Autodesk Inventor part; units mm, degrees
ref_plane "YZ Plane" through (0, 0, 0) normal (1, 0, 0) x (0, 1, 0)
ref_plane "XZ Plane" through (0, 0, 0) normal (0, 1, 0) x (-1, 0, 0)
ref_plane "XY Plane" through (0, 0, 0) normal (0, 0, 1) x (1, 0, 0)
sketch "Boceto1" plane through (0, 0, 0) normal (0, 0, 1) x (1, 0, 0)
  line L0 (0.1195, 0.0416) -> (6.4695, 0.0416)
  line L1 (6.4695, 0.0416) -> (6.4695, 19.0916)
  line L2 (6.4695, 19.0916) -> (0.1195, 19.0916)
  line L3 (0.1195, 19.0916) -> (0.1195, 0.0416)
  line L4 (6.4695, 0.0416) -> (20.6935, 0.0416)
  line L5 (20.6935, 0.0416) -> (20.6935, 26.2036)
  line L6 (20.6935, 26.2036) -> (6.4695, 26.2036)
  line L7 (6.4695, 26.2036) -> (6.4695, 0.0416)
  line L8 (20.6935, 0.0416) -> (30.3455, 0.0416)
  line L9 (30.3455, 0.0416) -> (30.3455, 22.3936)
  line L10 (30.3455, 22.3936) -> (20.6935, 22.3936)
  line L11 (20.6935, 22.3936) -> (20.6935, 0.0416)
  line L12 (30.3455, 0.0416) -> (44.5695, 0.0416)
  line L13 (44.5695, 0.0416) -> (44.5695, 26.2036)
  line L14 (44.5695, 26.2036) -> (30.3455, 26.2036)
  line L15 (30.3455, 26.2036) -> (30.3455, 0.0416)
  line L16 (44.5695, 0.0416) -> (50.9195, 0.0416)
  line L17 (50.9195, 0.0416) -> (50.9195, 19.0916)
  line L18 (50.9195, 19.0916) -> (44.5695, 19.0916)
  line L19 (44.5695, 19.0916) -> (44.5695, 0.0416)
  line L20 (0.1195, 0.0416) -> (50.9195, 0.0416)
  dimension "d2" = 19.05
  dimension "d3" = 26.162
  dimension "d4" = 9.652
  dimension "d5" = 50.8
  dimension "d6" = 14.224
  dimension "d7" = 6.35
  dimension "d8" = 3.81
revolve "Revolución1" add sketch "Boceto1" angle 360 about axis through (0.1195, 0.0416, 0) along (1, 0, 0)
sketch "Boceto2" plane through (0.1195, 0.0416, 0) normal (-1, 0, 0) x (0, 0, 1)
  circle A0 centre (0, -0.0416) radius 10.9883
extrude "Extrusión1" cut sketch "Boceto2" against normal blind 50.8
equation "\"d2\" = 0.5 * DistC"
equation "\"d3\" = 0.5 * DistA"
equation "\"d4\" = DistE"
equation "\"d5\" = DistB"
equation "\"d6\" = DistX"
equation "\"d7\" = DistD - DistX"
equation "\"d10\" = DistB"
equation "\"DistA\" = 52.324"
equation "\"DistB\" = 50.8"
equation "\"DistC\" = 38.1"
equation "\"DistD\" = 20.574"
equation "\"DistE\" = 9.652"
equation "\"DistX\" = 14.224"
properties part number "Pieza2-Tarea2"
Build history of the part. All positions in model axes, mm. A direction names the side the tool comes from. Round coordinates to 2 decimals unless told otherwise and drop trailing zeros. Order: outer loops, then holes, each group sorted by start corner. A loop starts at its lowest first (then second) coordinate and runs counter-clockwise, first axis right, second up. Notation, with made-up numbers: (2.5, 66) -> (51.5, 66) arc R19 cw to (51.5, 73) -> close; hole circle Ø11 at (-34, 6). An arc over 180 degrees is marked (long way). Answer in a Markdown table with one row per item.
1) Wall check: L1, parallel to X at y = 24.5, z = -1.5; L2, parallel to Y at x = 25, z = -0.5; L3, parallel to Z at x = 36, y = -0.5. Give the ranges that are in metal, low to high.
Values:
| item | result |
|---|---|
| L1 | 6.47 to 20.69, 30.35 to 44.57 |
| L2 | -22.3 to -10.98, 10.98 to 22.39 |
| L3 | -26.16 to -10.98, 10.98 to 26.16 |
2) Mould opens along Z. For faces 6 (the cylindrical face through (25.16, 3.3, 10.48)), 7 (the cylindrical face through (37.358, 24.995, -7.858)), 8 (the flat face through (0.12, 8, -8)) say: released by +Z, released by -Z, zero draft, split by the parting line, or undercut.
Values:
| item | result |
|---|---|
| face 6 | undercut |
| face 7 | split by the parting line |
| face 8 | zero draft |
3) Band-saw the part on B-B on y = 0. Give the cut face in (x, z).
Values:
| item | result |
|---|---|
| outline | (0.12, -19.05) -> (6.47, -19.05) -> (6.47, -26.16) -> (20.69, -26.16) -> (20.69, -22.35) -> (30.35, -22.35) -> (30.35, -26.16) -> (44.57, -26.16) -> (44.57, -19.05) -> (50.92, -19.05) -> (50.92, -10.99) -> (0.12, -10.99) -> close; (0.12, 10.99) -> (50.92, 10.99) -> (50.92, 19.05) -> (44.57, 19.05) -> (44.57, 26.16) -> (30.35, 26.16) -> (30.35, 22.35) -> (20.69, 22.35) -> (20.69, 26.16) -> (6.47, 26.16) -> (6.47, 19.05) -> (0.12, 19.05) -> close |
4) Band-saw the part on D-D on x = 16. Give the cut face in (y, z).
Values:
| item | result |
|---|---|
| outline | circle Ø52.32 at (0.04, 0); hole circle Ø21.98 at (0, 0) |
5) Band-saw the part on A-A on z = 0. Give the cut face in (x, y), and give its area (3 significant figures).
Values:
| item | result |
|---|---|
| outline | (0.12, -19.01) -> (6.47, -19.01) -> (6.47, -26.12) -> (20.69, -26.12) -> (20.69, -22.31) -> (30.35, -22.31) -> (30.35, -26.12) -> (44.57, -26.12) -> (44.57, -19.01) -> (50.92, -19.01) -> (50.92, -10.99) -> (0.12, -10.99) -> close; (0.12, 10.99) -> (50.92, 10.99) -> (50.92, 19.09) -> (44.57, 19.09) -> (44.57, 26.2) -> (30.35, 26.2) -> (30.35, 22.39) -> (20.69, 22.39) -> (20.69, 26.2) -> (6.47, 26.2) -> (6.47, 19.09) -> (0.12, 19.09) -> close |
| area | 1,290 mm2 |
6) Band-saw the part on C-C on y = -21. Give the cut face in (x, z).
Values:
| item | result |
|---|---|
| outline | (6.47, -15.55) -> (20.69, -15.55) -> (20.69, -7.54) -> (30.35, -7.54) -> (30.35, -15.55) -> (44.57, -15.55) -> (44.57, 15.55) -> (30.35, 15.55) -> (30.35, 7.54) -> (20.69, 7.54) -> (20.69, 15.55) -> (6.47, 15.55) -> close |
7) Pin check, flat tips, straight feed: P1, Ø3, axis at y = 8, z = -2.5, coming from the +X side; P2, Ø8, axis at y = 19.5, z = -9.5, coming from the -X side; P3, Ø6, axis at x = 32.5, z = -10, coming from the -Y side; P4, Ø3, axis at x = 28.5, y = 5, coming from the -Z side. Stop position of each tip, or through.
Values:
| item | result |
|---|---|
| P1 | through |
| P2 | x = 0.12 |
| P3 | y = -25.17 |
| P4 | z = -22.08 |
8) Which spindle directions (+Z, -Z, +X, -X, +Y, -Y) get a long thin tool onto all of the face, cutting with end or side? Do faces 1 (the cylindrical face through (13.482, 24.995, -7.858)), 2 (the cylindrical face through (3.25, 18.212, -5.722)), 3 (the flat face through (44.57, 1.9, -19.3)), 4 (the cylindrical face through (25.452, -17.696, 13.601)), 5 (the flat face through (50.92, 8, -8)). Say none if no direction does.
Values:
| item | result |
|---|---|
| face 1 | +X, -X |
| face 2 | -X |
| face 3 | +X |
| face 4 | none |
| face 5 | +Z, -Z, +X, +Y, -Y |
